from build123d import *

# Parameters (mm, degrees)
F0_W          = 60
F0_H          = 40
F1_DEPTH      = 80
F4_W          = 60
F4_H          = 40
F5_DEPTH      = 25
F5_DEPTH_BACK = 80
F7_E7_W       = 192.0395717025
F7_E7_H       = 176.2685924768
F8_DEPTH      = 68.6223879457
F9_W          = 146.8224227428
F9_H          = 227.745719254
F10_DEPTH     = 104.3368522078


with BuildPart() as f1:
    # F0 (on Top) → F1 (new body)
    with BuildSketch(Plane.XY):
        with Locations((10, -0.2545155585)):
            Rectangle(F0_W, F0_H)
    extrude(amount=F1_DEPTH)

    # F2 (on Front) → F3 (revolve)
    with BuildSketch(Plane.XZ):
        with BuildLine():
            ThreePointArc((89.4427191, 0), (76.0845213036, 47.0228201834), (40, 80))
            Line((40, 80), (40, 0))
            Line((40, 0), (89.4427191, 0))
        make_face()
        with BuildLine():
            Line((40, 0), (40, 80))
            ThreePointArc((40, 80), (-47.0228201834, 76.0845213036), (-89.4427191, 0))
            Line((-89.4427191, 0), (40, 0))
        make_face()
    revolve(axis=Axis((0, 0, 0), (1, 0, 0)))

    # F4 (on face) → F5 (cut, two sides)
    with BuildSketch(Plane.XY.offset(80)) as f5_sk:
        with Locations((10, -0.2545155585)):
            Rectangle(F4_W, F4_H)
    extrude(amount=F5_DEPTH, mode=Mode.SUBTRACT)
    extrude(f5_sk.sketch, amount=-F5_DEPTH_BACK, mode=Mode.SUBTRACT)

    # F7_E7 (on explicit) → F8 (cut)
    with BuildSketch(Plane(origin=(-31.5267369151, 88.1342962384, 105.66496104), x_dir=(0, 0, -1), z_dir=(-1, 0, 0))):
        with Locations((96.0197858512, 88.1342962384)):
            Rectangle(F7_E7_W, F7_E7_H)
    extrude(amount=F8_DEPTH, mode=Mode.SUBTRACT)

    # F9 (on Top) → F10 (cut)
    with BuildSketch(Plane.XY):
        with Locations((26.485607028, 2.56710127)):
            Rectangle(F9_W, F9_H)
    extrude(amount=-F10_DEPTH, mode=Mode.SUBTRACT)


solid = f1.part
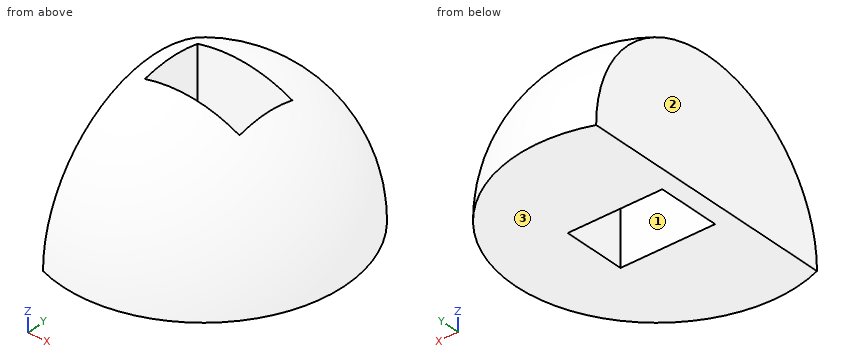
The model under review builds one solid part; all positions refer to its coordinate system, in mm. Face numbers are marked on the shaded views. Give positions to 0.01 mm unless a question says otherwise; leave off trailing zeros. Write each loop counter-clockwise with the first axis right and the second up, starting at its lowest first coordinate (ties: lowest second). Pieces come first, ordered by that corner, then holes.
1. Add section C-C, the plane z = 10.5. Write out the cut boundary in (x, y), plus the area to 3 significant figures.
2. Add section D-D, the plane z = 26. Write out the cut boundary in (x, y).
3. For P1, Ø1.5, axis at x = 35, y = -62.5, coming from the +Z side; P2, Ø20, axis at y = 7, z = 54.5, coming from the +X side; P3, Ø5, axis at x = -9.5, z = 72, coming from the -Y side; P4, Ø12, axis at y = -64.5, z = 72.5, coming from the -X side, all flat-tipped, find the tip position at first contact; note any pin that passes through.
4. Add section A-A, the plane y = -5. Write out the cut boundary in (x, z), plus the area to 3 significant figures.
5. Wall thickness on L1, parallel to X at y = -18.5, z = 68; L2, parallel to Y at x = 37.5, z = 7.5; L3, parallel to Y at x = -2, z = 5: over which ranges is each line inside the solid? List them lowest first.
6. Draft analysis for pull direction X (two halves, no side actions). For the marked faces 1, 2 and 3, state which applies: +X half, -X half, draft (parallel to the pull), parting line (faces both ways), or undercut.
7. Add section B-B, the plane x = -12. Write out the cut boundary in (y, z).
Worked answers:
1. outline: (-31.53, -83.04) arc R88.82 ccw (long way) to (-31.53, 83.04) - close; hole (-20, -20.25) - (40, -20.25) - (40, 19.75) - (-20, 19.75) - close
1. area: 15,500 mm2
2. outline: (-31.53, -79.56) arc R85.58 ccw (long way) to (-31.53, 79.56) - close; hole (-20, -20.25) - (40, -20.25) - (40, 19.75) - (-20, 19.75) - close
3. P1: stops at z = 54.55
3. P2: stops at x = 77.33
3. P3: stops at y = -55.52
3. P4: passes through
4. outline: (-31.53, 0) - (-20, 0) - (-20, 87.03) arc R89.3 ccw to (-31.53, 83.55) - close; (40, 0) - (89.3, 0) arc R89.3 ccw to (40, 79.84) - close
4. area: 3,800 mm2
5. L1: x = -31.53 to -20, 40 to 55.08
5. L2: y = -80.85 to -20.25, 19.75 to 80.85
5. L3: y = -89.28 to -20.25, 19.75 to 89.28
6. face 1: undercut
6. face 2: -X half
6. face 3: draft
7. outline: (-88.63, 0) - (-20.25, 0) - (-20.25, 86.29) arc R88.63 ccw to start; (19.75, 0) - (88.63, 0) arc R88.63 ccw to (19.75, 86.41) - close
